from build123d import *

# Parameters (mm, degrees)
TIP_CHAMFER_SIZE = 0.25
M3_TAPPED_HOLE_D = 2.5


with BuildPart() as part:
    # Body Sketch → Body Revolve (revolve)
    with BuildSketch(Plane.XY, mode=Mode.PRIVATE) as body_revolve_sk:
        Polygon((0, 0), (2.78, 0), (2.78, 3), (2.045, 3), (2.045, 4.53), (0, 4.53), align=None)
    revolve(body_revolve_sk.sketch.rotate(Axis((0, 4.53, 0), (0, -1, 0)), 180), axis=Axis((0, 4.53, 0), (0, -1, 0)))

    # Tip Chamfer
    tip_chamfer_edges = [part.edges().sort_by_distance(p)[0] for p in [
        (2.045, 4.53, 0),
    ]]
    chamfer(tip_chamfer_edges, length=TIP_CHAMFER_SIZE)

    # M3 Tapped Hole (through all)
    with Locations(Plane(origin=(0, 0, 0), x_dir=(-1, 0, 0), z_dir=(0, -1, 0))):
        with Locations((0, 0)):
            Hole(M3_TAPPED_HOLE_D / 2)


solid = part.part
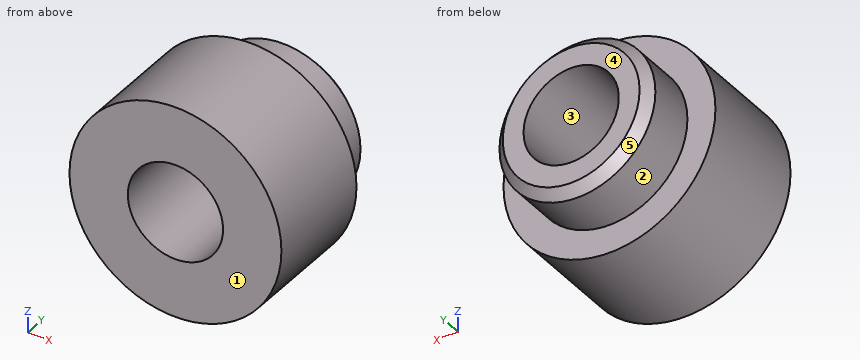
Can you work these out from the model? Positions are in its coordinate system, mm. Face numbers are marked on the shaded views. A direction names the side the tool comes from. Coordinates: 2 decimals unless noted, no trailing zeros. Order: outer loops, then holes, each group sorted by start corner. A loop starts at its lowest first (then second) coordinate and runs counter-clockwise, first axis right, second up. Notation, with made-up numbers: M -4.5,26.25 L 27.5,26.25 A18 ccw 27.5,39.25 Z; hole C 68.25,-35 d6. An arc over 180 degrees is marked long. Answer as CSV lines item,"result".
(1) Please list where these lines run through material, in increasing order: L1, parallel to Z at x = 0, y = 1.15; L2, parallel to X at y = 3.65, z = -0.85; L3, parallel to Z at x = -0.6, y = 0.65.
Geometry check:
L1,"-2.78 to -1.25, 1.25 to 2.78"
L2,"-1.86 to -0.92, 0.92 to 1.86"
L3,"-2.71 to -1.1, 1.1 to 2.71"
(2) I'm going to push a flat-ended pin straight in: pin 1 (1 mm diameter, centred on x = -1.5, y = 3, fed in from +Z). Where does the tip first touch, or does it pass through?
Geometry check:
pin 1,"z = 2.59"
(3) Suppose I cut it at C-C on y = 2.1. Please give me the cut outline in (x, z), plus the area to 3 significant figures.
Geometry check:
outline,"C 0,0 d5.56; hole C 0,0 d2.5"
area,"19.4 mm^2"
(4) Suppose I cut it at D-D on z = 2.3. Please give me the cut outline in (x, y), plus the area to 3 significant figures.
Geometry check:
outline,"M -1.56,0 L 1.56,0 L 1.56,3 L -1.56,3 Z"
area,"9.37 mm^2"
(5) Suppose I cut it at B-B on x = 0. Please give me the cut outline in (y, z) (3 decimals).
Geometry check:
outline,"M 0,-2.78 L 3,-2.78 L 3,-2.045 L 4.28,-2.045 L 4.53,-1.795 L 4.53,-1.25 L 0,-1.25 Z; M 0,1.25 L 4.53,1.25 L 4.53,1.795 L 4.28,2.045 L 3,2.045 L 3,2.78 L 0,2.78 Z"
(6) Suppose I cut it at A-A on z = 0. Please give me the cut outline in (x, y) (3 decimals), plus the area to 3 significant figures.
Geometry check:
outline,"M -2.78,0 L -1.25,0 L -1.25,4.53 L -1.795,4.53 L -2.045,4.28 L -2.045,3 L -2.78,3 Z; M 1.25,0 L 2.78,0 L 2.78,3 L 2.045,3 L 2.045,4.28 L 1.795,4.53 L 1.25,4.53 Z"
area,"11.6 mm^2"
(7) If we mould it in two halves opening along X, with no side actions, what happens to the marked faces 3, 4 and 5? For each: released by +X, released by -X, zero draft, split by the parting line, or undercut.
Geometry check:
face 3,"undercut"
face 4,"zero draft"
face 5,"split by the parting line"
(8) On a 3-axis mill with a long thin cutter (end or side, diameter ignored), from which of +Z, -Z, +X, -X, +Y, -Y can I reach the whole of each face in a straight line? I mean the marked faces 1 and 2. Say none if no direction works.
Geometry check:
face 1,"+Z, -Z, +X, -X, -Y"
face 2,"+Y"
